from build123d import *

# Parameters (mm, degrees)
F0_R      = 11
F1_DEPTH  = 14.5
F2_R      = 2.1
F3_DEPTH  = 3.5
F4_R      = 11
F5_DEPTH  = 3.5
F7_DEPTH  = 3.5
F8_R      = 6.5
F9_DEPTH  = 7.87
F10_R     = 0.2032
F11_DEPTH = 25


# Not quite as in the source:
# - a pattern or mirror of a feature is missing from the dataset's text; its kind, count and spacing are read off the source's solid


with BuildPart() as f1:
    # F0 (on Top) → F1 (new body)
    with BuildSketch(Plane.XY):
        Circle(F0_R)
    extrude(amount=F1_DEPTH)

    # F2 (on face) → F3 (join)
    with BuildSketch(Plane(origin=(0, 0, 0), x_dir=(1, 0, 0), z_dir=(0, 0, -1))):
        with BuildLine():
            Line((9.5262794416, 5.5), (3.0310889132, 16.75))
            ThreePointArc((3.0310889132, 16.75), (0, 18.5), (-3.0310889132, 16.75))
            Line((-3.0310889132, 16.75), (-9.5262794416, 5.5))
            ThreePointArc((-9.5262794416, 5.5), (0, 11), (9.5262794416, 5.5))
        make_face()
        with Locations((0, 15)):
            Circle(F2_R, mode=Mode.SUBTRACT)
        with BuildLine():
            ThreePointArc((9.5262794416, -5.5), (0, -11), (-9.5262794416, -5.5))
            Line((-9.5262794416, -5.5), (-3.0310889132, -16.75))
            ThreePointArc((-3.0310889132, -16.75), (0, -18.5), (3.0310889132, -16.75))
            Line((3.0310889132, -16.75), (9.5262794416, -5.5))
        make_face()
        with Locations((0, -15)):
            Circle(F2_R, mode=Mode.SUBTRACT)
    f3 = extrude(amount=-F3_DEPTH)

    # F3_copies: F3 across plane
    add(f3.mirror(Plane(origin=(0, 0, 0), x_dir=(0, 0, -1), z_dir=(-1, 0, 0))))

    # F4 (on face) → F5 (cut)
    with BuildSketch(Plane.XY.offset(3.5)):
        Circle(F4_R)
    extrude(amount=F5_DEPTH, mode=Mode.SUBTRACT)

    # F6 (on face) → F7 (join)
    with BuildSketch(Plane.XY.offset(3.5)):
        Polygon((9.5262794416, 5.5), (0, 11), (-9.5262794416, 5.5), (-9.5262794416, -5.5), (0, -11), (9.5262794416, -5.5), align=None)
    extrude(amount=F7_DEPTH)

    # F8 (on face) → F9 (cut)
    with BuildSketch(Plane(origin=(0, 0, 0), x_dir=(1, 0, 0), z_dir=(0, 0, -1))):
        Circle(F8_R)
    extrude(amount=-F9_DEPTH, mode=Mode.SUBTRACT)

    # F10 (on face) → F11 (join)
    with BuildSketch(Plane.XY.offset(14.5)):
        with Locations((6.7, 0)):
            Circle(F10_R)
        with Locations((6.7, 0.4318)):
            Circle(F10_R)
        with Locations((6.7, -0.4318)):
            Circle(F10_R)
    extrude(amount=F11_DEPTH)


solid = f1.part
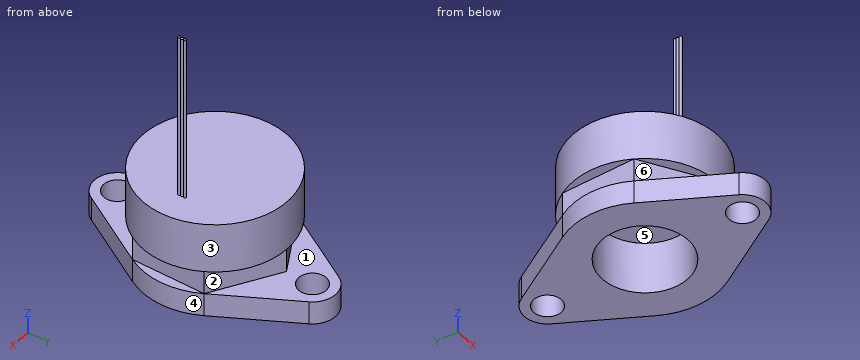
Here's how the part is built. I have some questions about the finished solid (model axes, mm). Face numbers are marked on the shaded views. A direction names the side the tool comes from. Give positions to 0.01 mm unless a question says otherwise; leave off trailing zeros. Order: outer loops, then holes, each group sorted by start corner. A loop starts at its lowest first (then second) coordinate and runs counter-clockwise, first axis right, second up. Notation, with made-up numbers: (25, -12) -> (29, -12) arc R24 ccw to (29, 11) -> close; hole circle Ø5 at (71, 32.5). An arc over 180 degrees is marked (long way). Use a Markdown table: item, result. Add a question column.
Item 1: I need wall thicknesses on line 1 (X direction, y = 0, z = 4); line 2 (Z direction, x = 5.25, y = -8.5); line 3 (Y direction, x = 2.25, z = 6). Which ranges of each line are inside material? Lowest first, please.
Item 2: For the marked faces 1, 2 and 3, which set-ups out of +Z, -Z, +X, -X, +Y, -Y let a thin tool reach every point of the face, with its end or its side?
Item 3: Imagine slicing it at C-C on x = -4.75. Please give me the cut outline in (y, z).
Item 4: Will these pins go through, and if not, where does the flat tip stop? pin 1 (6.5 mm diameter, centred on x = 1, y = -2, fed in from +Z); pin 2 (12 mm diameter, centred on x = -8.5, z = 5.5, fed in from +Y); pin 3 (4 mm diameter, centred on x = 8, z = 23.5, fed in from -Y) (3 decimals).
Item 5: Imagine slicing it at A-A on z = 5. Please give me the cut outline in (x, y).
Item 6: Imagine slicing it at B-B on y = 15. Please give me the cut outline in (x, z).
Item 7: If we mould it in two halves opening along Y, with no side actions, what happens to the marked faces 4, 5 and 6? For each: pulls with the +Y half, pulls with the -Y half, needs draft (parallel to the pull), parting line crosses it, or undercut.
Item 8: Imagine slicing it at D-D on y = 8.5. Please give me the cut outline in (x, z), plus the area to 3 significant figures.
Data:
| question | item | result |
|---|---|---|
| 1 | line 1 | x = -9.53 to -6.5, 6.5 to 9.53 |
| 1 | line 2 | z = 0 to 3.5, 7 to 14.5 |
| 1 | line 3 | y = -9.7 to -6.1, 6.1 to 9.7 |
| 2 | face 1 | +Y |
| 2 | face 2 | +X, +Y |
| 2 | face 3 | +Z |
| 3 | outline | (-13.77, 0) -> (-4.44, 0) -> (-4.44, 7.87) -> (4.44, 7.87) -> (4.44, 0) -> (13.77, 0) -> (13.77, 3.5) -> (8.26, 3.5) -> (8.26, 7) -> (9.92, 7) -> (9.92, 14.5) -> (-9.92, 14.5) -> (-9.92, 7) -> (-8.26, 7) -> (-8.26, 3.5) -> (-13.77, 3.5) -> close |
| 4 | pin 1 | stops at z = 14.5 |
| 4 | pin 2 | stops at y = 17.04 |
| 4 | pin 3 | stops at y = -0.635 |
| 5 | outline | (-9.53, -5.5) -> (0, -11) -> (9.53, -5.5) -> (9.53, 5.5) -> (0, 11) -> (-9.53, 5.5) -> close; hole circle Ø13 at (0, 0) |
| 6 | outline | (-4.04, 0) -> (-2.1, 0) -> (-2.1, 3.5) -> (-4.04, 3.5) -> close; (2.1, 0) -> (4.04, 0) -> (4.04, 3.5) -> (2.1, 3.5) -> close |
| 7 | face 4 | parting line crosses it |
| 7 | face 5 | undercut |
| 7 | face 6 | pulls with the -Y half |
| 8 | outline | (-7.79, 0) -> (7.79, 0) -> (7.79, 3.5) -> (4.33, 3.5) -> (4.33, 7) -> (6.98, 7) -> (6.98, 14.5) -> (-6.98, 14.5) -> (-6.98, 7) -> (-4.33, 7) -> (-4.33, 3.5) -> (-7.79, 3.5) -> close |
| 8 | area | 190 mm² |
